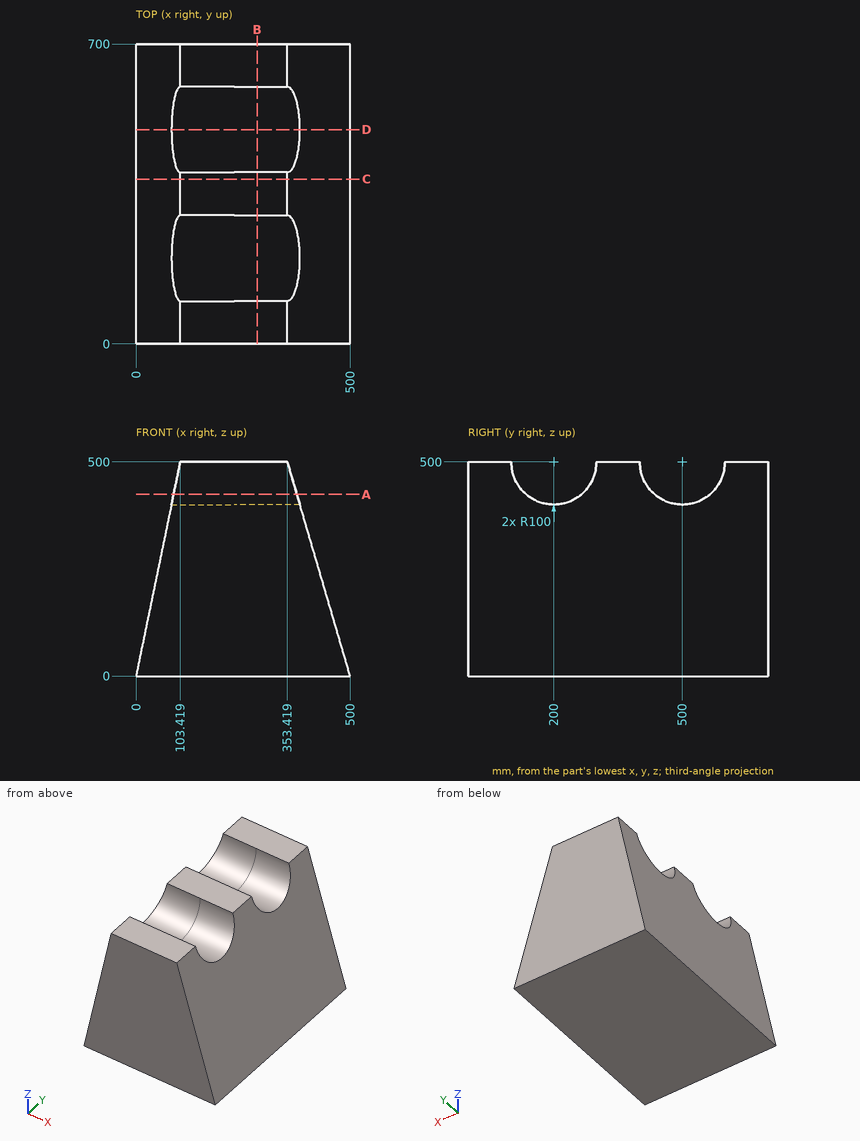
The figure shows three views and two pictorial views of one solid part (mm, origin at its lowest corner). Answer the questions. Coordinates: 2 decimals unless noted, no trailing zeros. Loops run counter-clockwise (first coordinate to the right, second up) from the corner with the lowest first, then second, coordinate; pieces in that order, holes last.
1) Find section B-B on x = 283. Write down the section's boundary in (y, z), then the cut area to 3 significant figures.
2) Flat-ended cylindrical pins translate along their axes: pin 1 Ø6 at (y, z) = (421, 417.5) entering from -X; pin 2 Ø4 at (y, z) = (339, 134) entering from -X; pin 3 Ø10 at (y, z) = (89.5, 155.5) entering from +X. Find the tip coordinate at first contact, or state that the pin passes through.
3) Find section C-C on y = 384.5. Write down the section's boundary in (x, z).
4) Find the intervals of material crossed by L1, parallel to X at y = 164, z = 400 (3 decimals); L2, parallel to Y at x = 350, z = 410.5; L3, parallel to X at y = 241, z = 44.5, in increasing order.
5) Find section D-D on y = 500. Write down the section's boundary in (x, z) (3 decimals).
6) Find section A-A on z = 424. Write down the section's boundary in (x, y), then the cut area to 3 significant figures.
Values:
1. outline: (0, 0) - (700, 0) - (700, 500) - (600, 500) arc R100 cw to (400, 500) - (300, 500) arc R100 cw to (100, 500) - (0, 500) - close
1. area: 319,000 mm2
2. pin 1: stops at x = 85.73
2. pin 2: stops at x = 27.3
2. pin 3: stops at x = 455.88
3. outline: (0, 0) - (500, 0) - (353.42, 500) - (103.42, 500) - close
4. L1: x = 82.735 to 382.735
4. L2: y = 0 to 155.39, 244.61 to 455.39, 544.61 to 700
4. L3: x = 9.2 to 486.95
5. outline: (0, 0) - (500, 0) - (382.735, 400) - (82.735, 400) - close
6. outline: (87.7, 0) - (375.7, 0) - (375.7, 135.01) - (87.7, 135.01) - close; (87.7, 264.99) - (375.7, 264.99) - (375.7, 435.01) - (87.7, 435.01) - close; (87.7, 564.99) - (375.7, 564.99) - (375.7, 700) - (87.7, 700) - close
6. area: 127,000 mm2
